Input: dimensioned drawing with shaded views. Units: mm. Origin: part minimum x, y, z. A direction names the side the tool comes from. Give positions to 0.01 mm unless a question says otherwise; leave off trailing zeros. Loops run counter-clockwise (first coordinate to the right, second up) from the corner with the lowest first, then second, coordinate; pieces in that order, holes last. Notation, with made-up numbers: (33, 31.5) -> (61, 31.5) arc R22 ccw to (61, 55.5) -> close; hole circle Ø10 at (20.5, 26). An arc over 180 degrees is marked (long way). Answer in a Markdown table with one row per item. Add a question column.
1) Section query A-A (y = 4). Return the cut outline in (x, z), plus the area to 3 significant figures.
2) Draft query along X for the marked faces 3, 4 and 5. Return one class per face: +X half, -X half, draft (parallel to the pull), parting line (faces both ways), or undercut.
3) Access query for the marked faces 1 and 2. Directions: +Z, -Z, +X, -X, +Y, -Y. A direction counts if a zero-diameter tool reaches every point of the face in a straight line with its end or side. Return the directions, or none.
4) Line query: line 1 (Z direction, x = 24.5, y = 7.25); line 2 (Z direction, x = 24.5, y = 10.75); line 3 (Z direction, x = 11.5, y = 9.25). Output: solid intervals per line, ascending. Write a range as from..to.
5) First-contact query: P1, Ø10, axis at x = 30, z = 13.5, coming from the -Y side; P2, Ø5, axis at x = 35, y = 7, coming from the -Z side; P3, Ø8, axis at y = 6.5, z = 11, coming from the -X side; P4, Ø3, axis at y = 4.5, z = 12.5, coming from the +X side. Flat tips, straight axial feed; report the tip coordinate or a pass-through.
6) Section query D-D (x = 11). Give the number of separate pieces and of enclosed holes in the cut face, plus the area to 3 significant figures.
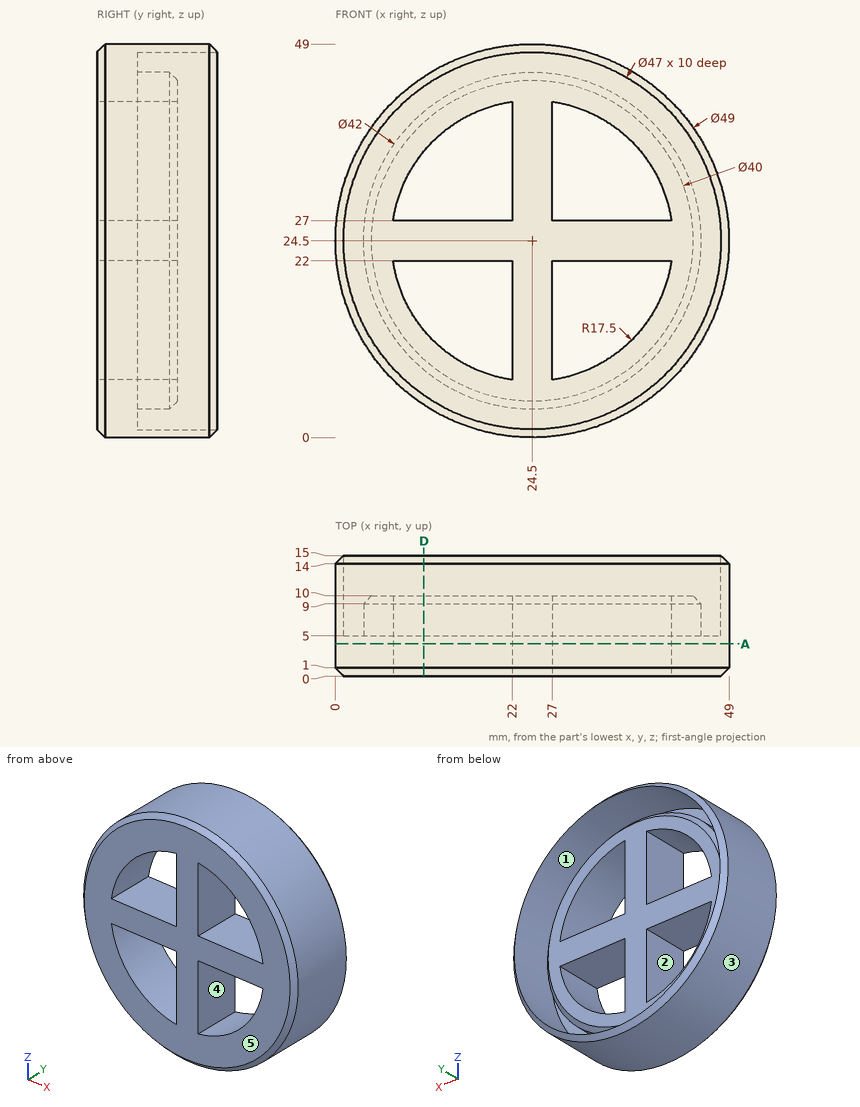
Evaluation:
| question | item | result |
|---|---|---|
| 1 | outline | circle Ø49 at (24.5, 24.5); hole (7.18, 22) arc R17.5 ccw to (22, 7.18) -> (22, 22) -> close; hole (7.18, 27) -> (22, 27) -> (22, 41.82) arc R17.5 ccw to start; hole (27, 7.18) arc R17.5 ccw to (41.82, 22) -> (27, 22) -> close; hole (27, 27) -> (41.82, 27) arc R17.5 ccw to (27, 41.82) -> close |
| 1 | area | 1,250 mm² |
| 2 | face 3 | parting line |
| 2 | face 4 | undercut |
| 2 | face 5 | draft |
| 3 | face 1 | +Y |
| 3 | face 2 | +Y, -Y |
| 4 | line 1 | 0..1, 3.5..45.5, 48..49 |
| 4 | line 2 | 0..1, 48..49 |
| 4 | line 3 | 3.73..4.92, 8.33..12.78, 22..27, 36.22..40.67, 44.08..45.27 |
| 5 | P1 | y = 0 |
| 5 | P2 | z = 1.34 |
| 5 | P3 | x = 1.92 |
| 5 | P4 | x = 46.64 |
| 6 | separate pieces | 3 |
| 6 | enclosed holes | 0 |
| 6 | area | 213 mm² |
